from build123d import *

# Parameters (mm, degrees)
ESQUISSE1_W             = 20
ESQUISSE1_H             = 40
BOSS_EXTRU_1_DEPTH      = 36
ESQUISSE2_W             = 20
ESQUISSE2_H             = 7
BOSS_EXTRU_2_DEPTH      = 11
ESQUISSE3_W             = 20
ESQUISSE3_H             = 7
ENL_V_MAT_EXTRU_1_DEPTH = 7
ESQUISSE4_R             = 2.5
BOSS_EXTRU_3_DEPTH      = 7
ESQUISSE5_R             = 2.5
ENL_V_MAT_EXTRU_2_DEPTH = 7
ESQUISSE6_R             = 2.5
ENL_V_MAT_EXTRU_3_DEPTH = 7


with BuildPart() as part:
    # Esquisse1 → Boss.-Extru.1 (new body)
    with BuildSketch(Plane.XY):
        with Locations((10, -20)):
            Rectangle(ESQUISSE1_W, ESQUISSE1_H)
    extrude(amount=BOSS_EXTRU_1_DEPTH)

    # Esquisse2 → Boss.-Extru.2 (add)
    with BuildSketch(Plane.XY.offset(36)):
        with Locations((10, 3.5)):
            Rectangle(ESQUISSE2_W, ESQUISSE2_H)
        with Locations((10, -43.5)):
            Rectangle(ESQUISSE2_W, ESQUISSE2_H)
    extrude(amount=-BOSS_EXTRU_2_DEPTH)

    # Esquisse3 → Enlèv. mat.-Extru.1 (cut)
    with BuildSketch(Plane.XY.offset(36)):
        with Locations((10, -43.5)):
            Rectangle(ESQUISSE3_W, ESQUISSE3_H)
        with Locations((10, 3.5)):
            Rectangle(ESQUISSE3_W, ESQUISSE3_H)
    extrude(amount=-ENL_V_MAT_EXTRU_1_DEPTH, mode=Mode.SUBTRACT)

    # Esquisse4 → Boss.-Extru.3 (add)
    with BuildSketch(Plane.XY.offset(36)):
        with Locations((10, -10)):
            Circle(ESQUISSE4_R)
    extrude(amount=BOSS_EXTRU_3_DEPTH)

    # Esquisse5 → Enlèv. mat.-Extru.2 (cut)
    with BuildSketch(Plane.XY.offset(29)):
        with Locations((4.5, -45)):
            Circle(ESQUISSE5_R)
        with Locations((15.5, -45)):
            Circle(ESQUISSE5_R)
    extrude(amount=-ENL_V_MAT_EXTRU_2_DEPTH, mode=Mode.SUBTRACT)

    # Esquisse6 → Enlèv. mat.-Extru.3 (cut)
    with BuildSketch(Plane.XY.offset(29)):
        with Locations((4.5, 5)):
            Circle(ESQUISSE6_R)
        with Locations((15.5, 5)):
            Circle(ESQUISSE6_R)
    extrude(amount=-ENL_V_MAT_EXTRU_3_DEPTH, mode=Mode.SUBTRACT)


solid = part.part
Verification items for the finished model (mm, model axes). A direction names the side the tool comes from. Give positions to 0.01 mm unless a question says otherwise; leave off trailing zeros. Write each loop counter-clockwise with the first axis right and the second up, starting at its lowest first coordinate (ties: lowest second). Pieces come first, ordered by that corner, then holes. Notation, with made-up numbers: M -37.75,88.25 L -10.75,88.25 A17 cw -10.75,104.25 Z; hole C -39,74.5 d7. An arc over 180 degrees is marked long. Write item = value, one per line.
(1) Sectioned sample at D-D (y = -1.5). Record the cut outline in (x, z).
Found:
outline = M 0,0 L 20,0 L 20,36 L 0,36 Z
(2) Draft check along X on faces 6 (the face through (1, -47, 27)), 7 (the face through (9.46, -12.44, 39.45)), 8 (the face through (15.4, 2.5, 27)). Enter one of: released by +X, released by -X, zero draft, split by the parting line, or undercut.
Found:
face_6 = zero draft
face_7 = split by the parting line
face_8 = undercut
(3) Sectioned sample at C-C (z = 27). Record the cut outline in (x, y), then the cut area to 3 significant figures.
Found:
outline = M 0,-47 L 3,-47 A2.5 cw long 6,-47 L 14,-47 A2.5 cw long 17,-47 L 20,-47 L 20,7 L 17,7 A2.5 cw long 14,7 L 6,7 A2.5 cw long 3,7 L 0,7 Z
area = 1,010 mm2
(4) Sectioned sample at B-B (x = 10). Record the cut outline in (y, z).
Found:
outline = M -47,25 L -40,25 L -40,0 L 0,0 L 0,25 L 7,25 L 7,29 L 0,29 L 0,36 L -7.5,36 L -7.5,43 L -12.5,43 L -12.5,36 L -40,36 L -40,29 L -47,29 Z
(5) Access from +Z, -Z, +X, -X, +Y, -Y to the whole of each face (thin tool, end or side, straight path). Record for faces 1 (the face through (10, 3, 29)), 2 (the face through (10, -43, 29)), 3 (the face through (4.6, -42.5, 27)), 4 (the face through (10, 3, 25)), 5 (the face through (10, -43, 25)).
Found:
face_1 = +Z, +X, -X, +Y
face_2 = +Z, +X, -X, -Y
face_3 = +Z, -Z
face_4 = -Z, +X, -X, +Y
face_5 = -Z, +X, -X, -Y
(6) Go/stop test with flat-tipped pins: pin 1 Ø6 at (x, y) = (4.5, 5) entering from +Z; pin 2 Ø1 at (x, y) = (17.5, -38) entering from +Z; pin 3 Ø3.5 at (x, z) = (5.5, 34) entering from +Y; pin 4 Ø4.5 at (x, y) = (4.5, -45) entering from -Z. Record where each tip stops, or that it passes through.
Found:
pin_1 = 29
pin_2 = 36
pin_3 = 0
pin_4 = through
(7) Sectioned sample at A-A (y = 5). Record the cut outline in (x, z).
Found:
outline = M 0,25 L 2,25 L 2,29 L 0,29 Z; M 7,25 L 13,25 L 13,29 L 7,29 Z; M 18,25 L 20,25 L 20,29 L 18,29 Z
(8) Material ranges on line 1 (X direction, y = -45, z = 28); line 2 (Z direction, x = 3, y = -30.5); line 3 (Y direction, x = 4.5, z = 26.9), recorded low to high.
Found:
line_1 = 0 to 2, 7 to 13, 18 to 20
line_2 = 0 to 36
line_3 = -42.5 to 2.5
